Verification items for the finished model (mm, model axes). A direction names the side the tool comes from. Round coordinates to 2 decimals unless told otherwise and drop trailing zeros. Order: outer loops, then holes, each group sorted by start corner. A loop starts at its lowest first (then second) coordinate and runs counter-clockwise, first axis right, second up. Notation, with made-up numbers: (4, 55) -> (39, 55) arc R12 cw to (39, 66) -> close; hole circle Ø8 at (18, 41.5). An arc over 180 degrees is marked (long way). Put each result on its own line as item: value.
from build123d import *

# Parameters (mm, degrees)
SKETCH1_W                  = 30
SKETCH1_H                  = 30
SKETCH1_R                  = 1.6
SKETCH1_W_2                = 70
SKETCH1_H_2                = 12
BOSS_EXTRUDE1_DEPTH        = 6
SKETCH1_3_W                = 30
SKETCH1_3_H                = 30
SKETCH1_3_R                = 1.6
BOSS_EXTRUDE2_DEPTH        = 22.33
CUT_EXTRUDE1_DEPTH         = 22.5
SKETCH3_R                  = 2.55
CUT_EXTRUDE2_DEPTH         = 8
CUT_EXTRUDE3_DEPTH         = 4.5
SKETCH6_R                  = 5
CUT_EXTRUDE5_DEPTH         = 8.6
SKETCH7_R                  = 1.6
CUT_EXTRUDE6_DEPTH         = 101.740403513
SKETCH8_R                  = 2.85
CUT_EXTRUDE7_DEPTH         = 18
BOSS_EXTRUDE3_START        = 2.43
SKETCH9_R                  = 3.4
SKETCH9_R_2                = 2.55
BOSS_EXTRUDE3_DEPTH        = 2.43
CHAMFER1_SIZE              = 1.2
FILLET3_R                  = 4
CHAMFER2_SIZE              = 0.8
CUT_EXTRUDE8_DEPTH         = 3
CHAMFER3_SIZE              = 0.8
LPATTERN1_COUNT            = 3
LPATTERN1_PITCH            = 25
CHAMFER3_OF_LPATTERN1_SIZE = 0.8


with BuildPart() as part:
    # Sketch1 → Boss-Extrude1 (new body)
    # profile 1 of 2: a face of its own
    with BuildSketch(Plane.XY):
        with Locations((10, 10)):
            Rectangle(SKETCH1_W, SKETCH1_H)
        with Locations((20, 0)):
            Circle(SKETCH1_R, mode=Mode.SUBTRACT)
        with Locations((20, 20)):
            Circle(SKETCH1_R, mode=Mode.SUBTRACT)
        with Locations((0, 20)):
            Circle(SKETCH1_R, mode=Mode.SUBTRACT)
        Circle(SKETCH1_R, mode=Mode.SUBTRACT)
    # profile 2 of 2: a face of its own
    with BuildSketch(Plane.XY):
        with Locations((60, 10)):
            Rectangle(SKETCH1_W_2, SKETCH1_H_2)
    extrude(amount=BOSS_EXTRUDE1_DEPTH)

    # Sketch1_3 → Boss-Extrude2 (add)
    with BuildSketch(Plane.XY):
        with Locations((10, 10)):
            Rectangle(SKETCH1_3_W, SKETCH1_3_H)
        with Locations((20, 0)):
            Circle(SKETCH1_3_R, mode=Mode.SUBTRACT)
        with Locations((20, 20)):
            Circle(SKETCH1_3_R, mode=Mode.SUBTRACT)
        with Locations((0, 20)):
            Circle(SKETCH1_3_R, mode=Mode.SUBTRACT)
        Circle(SKETCH1_3_R, mode=Mode.SUBTRACT)
    extrude(amount=BOSS_EXTRUDE2_DEPTH)

    # Sketch2 → Cut-Extrude1 (cut)
    with BuildSketch(Plane(origin=(25, 0, 0), x_dir=(0, 0, -1), z_dir=(1, 0, 0))):
        with BuildLine():
            Line((-6.54075, 16.488632043), (-9.2445, 16.488632043))
            Line((-9.2445, 16.488632043), (-10.381879417, 16.288081364))
            ThreePointArc((-10.381879417, 16.288081364), (-11.49719937, 14.886920062), (-13.024482689, 15.822119108))
            Line((-13.024482689, 15.822119108), (-14.11125, 15.630492709))
            Line((-14.11125, 15.630492709), (-14.11125, 4.368771376))
            Line((-14.11125, 4.368771376), (-13.024482689, 4.177144977))
            ThreePointArc((-13.024482689, 4.177144977), (-11.49719937, 5.112344024), (-10.381879417, 3.711182721))
            Line((-10.381879417, 3.711182721), (-9.2445, 3.510632043))
            Line((-9.2445, 3.510632043), (-6.54075, 3.510632043))
            Line((-6.54075, 3.510632043), (-6, 4.051382043))
            Line((-6, 4.051382043), (-6, 15.947882043))
            Line((-6, 15.947882043), (-6.54075, 16.488632043))
        make_face()
    extrude(amount=-CUT_EXTRUDE1_DEPTH, mode=Mode.SUBTRACT)

    # Sketch3 → Cut-Extrude2 (cut)
    with BuildSketch(Plane.XY.offset(22.33)):
        with Locations((10, 10)):
            Circle(SKETCH3_R)
    extrude(amount=-CUT_EXTRUDE2_DEPTH, mode=Mode.SUBTRACT)

    # Sketch5 → Cut-Extrude3 (cut)
    with BuildSketch(Plane(origin=(0, 0, 14.11125), x_dir=(-1, 0, 0), z_dir=(0, 0, -1))):
        Polygon((-5.32346282, 10), (-7.66173141, 14.05), (-12.33826859, 14.05), (-14.67653718, 10), (-12.33826859, 5.95), (-7.66173141, 5.95), align=None)
    extrude(amount=-CUT_EXTRUDE3_DEPTH, mode=Mode.SUBTRACT)

    # Sketch6 → Cut-Extrude5 (cut)
    with BuildSketch(Plane(origin=(0, 0, 0), x_dir=(-1, 0, 0), z_dir=(0, 0, -1))):
        with Locations((-10, 10)):
            Circle(SKETCH6_R)
    extrude(amount=-CUT_EXTRUDE5_DEPTH, mode=Mode.SUBTRACT)

    # Sketch7 → Cut-Extrude6 (cut, through all)
    with BuildSketch(Plane(origin=(0, 0, 0), x_dir=(-1, 0, 0), z_dir=(0, 0, -1))):
        with BuildLine():
            ThreePointArc((-90.1, 10), (-88.5, 8.4), (-86.9, 10))
            Line((-86.9, 10), (-90.1, 10))
        make_face()
        with BuildLine():
            Line((-90.1, 10), (-86.9, 10))
            ThreePointArc((-86.9, 10), (-88.5, 11.6), (-90.1, 10))
        make_face()
        with Locations((-63.5, 10)):
            Circle(SKETCH7_R)
        with Locations((-38.5, 10)):
            Circle(SKETCH7_R)
    extrude(amount=-CUT_EXTRUDE6_DEPTH, mode=Mode.SUBTRACT)

    # Sketch8 → Cut-Extrude7 (cut)
    with BuildSketch(Plane.XY.offset(22.33)):
        with Locations((20, 20)):
            Circle(SKETCH8_R)
        with Locations((20, 0)):
            Circle(SKETCH8_R)
        Circle(SKETCH8_R)
        with Locations((0, 20)):
            Circle(SKETCH8_R)
    extrude(amount=-CUT_EXTRUDE7_DEPTH, mode=Mode.SUBTRACT)

    # Sketch9 → Boss-Extrude3 (add)
    with BuildSketch(Plane.XY.offset(22.33).offset(BOSS_EXTRUDE3_START)):
        with Locations(Location((10, 10, 0), (0, 0, 180))):
            Circle(SKETCH9_R)
        with Locations((10, 10)):
            Circle(SKETCH9_R_2, mode=Mode.SUBTRACT)
    extrude(amount=-BOSS_EXTRUDE3_DEPTH)

    # Chamfer1
    chamfer1_edges = [part.edges().sort_by_distance(p)[0] for p in [
        (13.4, 10, 22.33),
    ]]
    chamfer(chamfer1_edges, length=CHAMFER1_SIZE)

    # Fillet3
    fillet3_edges = [part.edges().sort_by_distance(p)[0] for p in [
        (-5, -5, 11.165),
        (-5, 25, 11.165),
        (25, 25, 11.165),
        (25, 16, 3),
        (95, 16, 3),
        (95, 4, 3),
        (25, 4, 3),
        (25, -5, 11.165),
    ]]
    fillet(fillet3_edges, radius=FILLET3_R)

    # Chamfer2
    chamfer2_edges = [part.edges().sort_by_distance(p)[0] for p in [
        (-2.85, 20, 22.33),
        (-2.85, 0, 22.33),
        (17.15, 0, 22.33),
        (17.15, 20, 22.33),
    ]]
    chamfer(chamfer2_edges, length=CHAMFER2_SIZE)

    # Sketch10 → Cut-Extrude8 (cut)
    with BuildSketch(Plane(origin=(0, 0, 0), x_dir=(-1, 0, 0), z_dir=(0, 0, -1))):
        Polygon((-85.266838493, 10), (-86.883419246, 12.8), (-90.116580754, 12.8), (-91.733161507, 10), (-90.116580754, 7.2), (-86.883419246, 7.2), align=None)
    cut_extrude8 = extrude(amount=-CUT_EXTRUDE8_DEPTH, mode=Mode.SUBTRACT)

    # Chamfer3
    chamfer3_edges = [part.edges().sort_by_distance(p)[0] for p in [
        (86.075128869, 8.6, 0),
        (86.075128869, 11.4, 0),
        (88.5, 12.8, 0),
        (90.924871131, 11.4, 0),
        (90.924871131, 8.6, 0),
        (88.5, 7.2, 0),
    ]]
    chamfer(chamfer3_edges, length=CHAMFER3_SIZE)

    # LPattern1: Cut-Extrude8 ×3
    with Locations(*[(-i * LPATTERN1_PITCH, 0, 0) for i in range(1, LPATTERN1_COUNT)]):
        add(cut_extrude8, mode=Mode.SUBTRACT)

    # Chamfer3 of LPattern1
    chamfer3_of_lpattern1_edges = [part.edges().sort_by_distance(p)[0] for p in [
        (61.075128869, 8.6, 0),
        (61.075128869, 11.4, 0),
        (63.5, 12.8, 0),
        (65.924871131, 11.4, 0),
        (65.924871131, 8.6, 0),
        (63.5, 7.2, 0),
        (36.075128869, 8.6, 0),
        (36.075128869, 11.4, 0),
        (38.5, 12.8, 0),
        (40.924871131, 11.4, 0),
        (40.924871131, 8.6, 0),
        (38.5, 7.2, 0),
    ]]
    chamfer(chamfer3_of_lpattern1_edges, length=CHAMFER3_OF_LPATTERN1_SIZE)


solid = part.part
Item 1: Section check B-B on z = 20.5. Record the boundary of the cut face in (x, y).
Check sheet entries:
outline: (-5, -1) arc R4 ccw to (-1, -5) -> (21, -5) arc R4 ccw to (25, -1) -> (25, 21) arc R4 ccw to (21, 25) -> (-1, 25) arc R4 ccw to (-5, 21) -> close; hole circle Ø5.7 at (0, 0); hole circle Ø5.7 at (0, 20); hole circle Ø5.1 at (10, 10); hole circle Ø5.7 at (20, 0); hole circle Ø5.7 at (20, 20)
Item 2: Gauge pin test, flat ends, axial feed: pin 1 Ø1.8 at (x, z) = (88, 2) entering from -Y; pin 2 Ø1.1 at (x, z) = (39, 2) entering from +Y; pin 3 Ø8 at (y, z) = (4.5, 9.5) entering from +X. Record the tip position at first contact, or that the pin passes through.
Check sheet entries:
pin 1: stops at y = 4
pin 2: stops at y = 16
pin 3: stops at x = 94.68
Item 3: Section check A-A on x = 38.5. Record the boundary of the cut face in (y, z), then the cut area to 3 significant figures.
Check sheet entries:
outline: (4, 0) -> (6.4, 0) -> (7.2, 0.8) -> (7.2, 3) -> (8.4, 3) -> (8.4, 6) -> (4, 6) -> close; (11.6, 3) -> (12.8, 3) -> (12.8, 0.8) -> (13.6, 0) -> (16, 0) -> (16, 6) -> (11.6, 6) -> close
area: 45.0 mm^2
Item 4: Material ranges on L1, parallel to Y at x = 0, z = 16.5; L2, parallel to Y at x = 38.5, z = 4.55; L3, parallel to X at y = 1.75, z = 6.75, recorded low to high. Write a range as [from, to].
Check sheet entries:
L1: y = [-5, -2.85], [2.85, 17.15], [22.85, 25]
L2: y = [4, 8.4], [11.6, 16]
L3: x = [-5, -2.25], [2.25, 17.75], [22.25, 25]
Item 5: Release check for a two-part mould opening along X. For faces 3 (the flat face through (62, 11, 3)), 4 (the cylindrical face through (23.797, -3.859, 11.321)), 5 (the flat face through (-5, 10, 11)) record: +X half, -X half, draft (parallel to the pull), parting line (faces both ways), or undercut.
Check sheet entries:
face 3: undercut
face 4: +X half
face 5: -X half
Item 6: Tool access check on faces 1 (the cylindrical face through (26.141, 2.797, 3.042)), 2 (the flat face through (91.28, 8.43, 0.41)). Record the directions out of +Z, -Z, +X, -X, +Y, -Y that give a thin tool (end or side, any length) a straight path to the whole face; none if there is none.
Check sheet entries:
face 1: +Z, -Z, +X, -Y
face 2: -Z
Item 7: Section check C-C on z = 16.25. Record the boundary of the cut face in (x, y), then the cut area to 3 significant figures.
Check sheet entries:
outline: (-5, -1) arc R4 ccw to (-1, -5) -> (21, -5) arc R4 ccw to (25, -1) -> (25, 21) arc R4 ccw to (21, 25) -> (-1, 25) arc R4 ccw to (-5, 21) -> close; hole circle Ø5.7 at (0, 0); hole circle Ø5.7 at (0, 20); hole (5.32, 10) -> (7.66, 5.95) -> (12.34, 5.95) -> (14.68, 10) -> (12.34, 14.05) -> (7.66, 14.05) -> close; hole circle Ø5.7 at (20, 0); hole circle Ø5.7 at (20, 20)
area: 727 mm^2
